```python
from build123d import *

# Parameters (mm, degrees)
F1_DEPTH = 10


with BuildPart() as f1:
    # F0 (on Front) → F1 (new body)
    with BuildSketch(Plane.XZ):
        with BuildLine():
            Line((148.27354, -200.430762), (99.685095, -7.929801))
            ThreePointArc((99.685095, -7.929801), (-28.245338, 95.928103), (-79.482166, -60.684308))
            Line((-79.482166, -60.684308), (-75.50395, -65.567931))
            Line((-75.50395, -65.567931), (55.654565, -226.576947))
            ThreePointArc((55.654565, -226.576947), (61.376545, -249.803158), (77.232841, -267.713373))
            Line((77.232841, -267.713373), (295.671613, -418.635733))
            ThreePointArc((295.671613, -418.635733), (332.558426, -414.834083), (325.084536, -378.51287))
            Line((325.084536, -378.51287), (155.36982, -221.248394))
            ThreePointArc((155.36982, -221.248394), (152.980519, -210.444555), (148.27354, -200.430762))
        make_face()
        with BuildLine():
            Line((-75.50395, -65.567931), (-79.482166, -60.684308))
            ThreePointArc((-79.482166, -60.684308), (-77.531519, -63.15745), (-75.50395, -65.567931))
        make_face()
    extrude(amount=F1_DEPTH)


solid = f1.part
```
The model under review builds one solid part; all positions refer to its coordinate system, in mm. Give positions to 0.01 mm unless a question says otherwise; leave off trailing zeros. Write each loop counter-clockwise with the first axis right and the second up, starting at its lowest first coordinate (ties: lowest second). Pieces come first, ordered by that corner, then holes. Notation, with made-up numbers: (38.5, 48) - (74.5, 48) arc R28 ccw to (74.5, 87) - close; hole circle Ø9 at (-22, 89). An arc over 180 degrees is marked (long way). Answer in a Markdown table with one row per item. Add a question column.
1. We need section A-A on y = -3.5. Write out the cut boundary in (x, z), then the cut area to 3 significant figures.
2. We need section B-B on x = 247. Write out the cut boundary in (y, z).
3. We need section C-C on z = 0. Write out the cut boundary in (x, y).
4. Insertion check: P1, Ø2, axis at x = 93, y = -3.5, coming from the -Z side; P2, Ø2, axis at y = -6.5, z = -52, coming from the -X side; P3, Ø6, axis at y = -8.5, z = -120, coming from the +X side. Each pin has a flat end and moves straight along its axis. Give the tip position at first contact, or say it passes through.
5. Wall thickness on line 1 along Z through (x, y) = (198, -8); line 2 along Z through (x, y) = (-5.5, -5); line 3 along X through (y, z) = (-4.5, -6): over which ranges is each line inside the solid? List them lowest first. Write a range as [from, to].
Ans:
| question | item | result |
|---|---|---|
| 1 | outline | (-79.48, -60.68) arc R100 ccw to (-75.5, -65.57) - (55.65, -226.58) arc R50 ccw to (77.23, -267.71) - (295.67, -418.64) arc R25 ccw (long way) to (325.08, -378.51) - (155.37, -221.25) arc R50 ccw to (148.27, -200.43) - (99.69, -7.93) arc R100 ccw (long way) to start |
| 1 | area | 71,800 mm^2 |
| 2 | outline | (-10, -385.01) - (0, -385.01) - (0, -306.16) - (-10, -306.16) - close |
| 3 | outline | (-100, -10) - (100, -10) - (100, 0) - (-100, 0) - close |
| 4 | P1 | stops at z = -279.3 |
| 4 | P2 | stops at x = -86.02 |
| 4 | P3 | stops at x = 128.73 |
| 5 | line 1 | z = [-351.15, -260.75] |
| 5 | line 2 | z = [-151.5, 99.85] |
| 5 | line 3 | x = [-99.82, 99.82] |
